Input: part model. Units: mm. Frame: model coordinates. Face numbers are marked on the shaded views. A direction names the side the tool comes from. Coordinates: 2 decimals unless noted, no trailing zeros. Order: outer loops, then holes, each group sorted by start corner. A loop starts at its lowest first (then second) coordinate and runs counter-clockwise, first axis right, second up. Notation, with made-up numbers: (-9, -18) -> (18, -18) arc R28 cw to (18, 20) -> close; hole circle Ø2 at (4.5, 7.25). An arc over 180 degrees is marked (long way). Answer as CSV lines item,"result".
from build123d import *

# Parameters (mm, degrees)
BOSS_EXTRU_1_START             = 0.6
ESQUISSE1_R                    = 47
ESQUISSE1_R_2                  = 20
BOSS_EXTRU_1_DEPTH             = 3
ESQUISSE2_R                    = 34.05
ESQUISSE2_R_2                  = 31.05
BOSS_EXTRU_2_DEPTH             = 8
CHANFREIN1_SIZE                = 0.5
TROU_TARAUD_M4X0_71_AT_2_COUNT = 2
TROU_TARAUD_M4X0_71_AT_2_PITCH = 12.5
TROU_TARAUD_M4X0_71_AT_3_COUNT = 2
TROU_TARAUD_M4X0_71_AT_3_PITCH = 82
TROU_TARAUD_M4X0_71_AT_4_COUNT = 2
TROU_TARAUD_M4X0_71_AT_4_PITCH = 82.947272408
TROU_TARAUD_M4X0_71_AT_5_COUNT = 2
TROU_TARAUD_M4X0_71_AT_5_PITCH = 49.143921292
TROU_TARAUD_M4X0_71_AT_6_COUNT = 2
TROU_TARAUD_M4X0_71_AT_6_PITCH = 58.652578801
TROU_TARAUD_M4X0_71_AT_7_COUNT = 2
TROU_TARAUD_M4X0_71_AT_7_PITCH = 66.821590822
TROU_TARAUD_M4X0_71_AT_8_COUNT = 2
TROU_TARAUD_M4X0_71_AT_8_PITCH = 58.652578801
TROU_TARAUD_M6X1_01_AT_2_COUNT = 2
TROU_TARAUD_M6X1_01_AT_2_PITCH = 20.705523608
TROU_TARAUD_M6X1_01_AT_3_COUNT = 2
TROU_TARAUD_M6X1_01_AT_3_PITCH = 56.568542495
TROU_TARAUD_M6X1_01_AT_4_COUNT = 2
TROU_TARAUD_M6X1_01_AT_4_PITCH = 69.282032303
TROU_TARAUD_M6X1_01_AT_5_COUNT = 2
TROU_TARAUD_M6X1_01_AT_5_PITCH = 80
TROU_TARAUD_M6X1_01_AT_6_COUNT = 2
TROU_TARAUD_M6X1_01_AT_6_PITCH = 77.274066103
TROU_TARAUD_M6X1_01_AT_7_COUNT = 2
TROU_TARAUD_M6X1_01_AT_7_PITCH = 56.568542495
TROU_TARAUD_M6X1_01_AT_8_COUNT = 2
TROU_TARAUD_M6X1_01_AT_8_PITCH = 40
D_GAGEMENT_M31_D               = 3.4


with BuildPart() as part:
    # Esquisse1 → Boss.-Extru.1 (new body)
    with BuildSketch(Plane.XY.offset(BOSS_EXTRU_1_START)):
        Circle(ESQUISSE1_R)
        Circle(ESQUISSE1_R_2, mode=Mode.SUBTRACT)
    extrude(amount=BOSS_EXTRU_1_DEPTH)

    # Esquisse2 → Boss.-Extru.2 (add)
    with BuildSketch(Plane(origin=(0, 0, 0.6), x_dir=(-1, 0, 0), z_dir=(0, 0, -1))):
        with Locations(Location((0, 0, 0), (0, 0, 180))):
            Circle(ESQUISSE2_R)
        Circle(ESQUISSE2_R_2, mode=Mode.SUBTRACT)
    extrude(amount=BOSS_EXTRU_2_DEPTH)

    # Chanfrein1
    chanfrein1_edges = [part.edges().sort_by_distance(p)[0] for p in [
        (-34.05, 0, -7.4),
        (31.05, 0, -7.4),
    ]]
    chamfer(chanfrein1_edges, length=CHANFREIN1_SIZE)

    # Esquisse15 → Trou taraudé M4x0.71 (revolve, cut)
    with BuildSketch(Plane(origin=(6.25, 41, 3.6), x_dir=(0, -1, 0), z_dir=(1, 0, 0))):
        Polygon((0, 0), (0, 3), (2.125, 3), (1.65, 2.525), (1.65, 0.475), (2.125, 0), align=None)
    trou_taraud_m4x0_71 = revolve(axis=Axis((6.25, 41, 9.95), (0, 0, -1)), mode=Mode.SUBTRACT)

    # Trou taraudé M4x0.71 at 2: Trou taraudé M4x0.71 ×2
    with Locations(*[(-i * TROU_TARAUD_M4X0_71_AT_2_PITCH, 0, 0) for i in range(1, TROU_TARAUD_M4X0_71_AT_2_COUNT)]):
        add(trou_taraud_m4x0_71, mode=Mode.SUBTRACT)

    # Trou taraudé M4x0.71 at 3: Trou taraudé M4x0.71 ×2
    with Locations(*[(0, -i * TROU_TARAUD_M4X0_71_AT_3_PITCH, 0) for i in range(1, TROU_TARAUD_M4X0_71_AT_3_COUNT)]):
        add(trou_taraud_m4x0_71, mode=Mode.SUBTRACT)

    # Trou taraudé M4x0.71 at 4: Trou taraudé M4x0.71 ×2
    with Locations(*[Vector(-0.15069814397812628, -0.9885798244965087, 0) * (i * TROU_TARAUD_M4X0_71_AT_4_PITCH) for i in range(1, TROU_TARAUD_M4X0_71_AT_4_COUNT)]):
        add(trou_taraud_m4x0_71, mode=Mode.SUBTRACT)

    # Trou taraudé M4x0.71 at 5: Trou taraudé M4x0.71 ×2
    with Locations(*[Vector(0.7071067811865477, -0.7071067811865474, 0) * (i * TROU_TARAUD_M4X0_71_AT_5_PITCH) for i in range(1, TROU_TARAUD_M4X0_71_AT_5_COUNT)]):
        add(trou_taraud_m4x0_71, mode=Mode.SUBTRACT)

    # Trou taraudé M4x0.71 at 6: Trou taraudé M4x0.71 ×2
    with Locations(*[Vector(0.5924718181265287, -0.8055911771648481, 0) * (i * TROU_TARAUD_M4X0_71_AT_6_PITCH) for i in range(1, TROU_TARAUD_M4X0_71_AT_6_COUNT)]):
        add(trou_taraud_m4x0_71, mode=Mode.SUBTRACT)

    # Trou taraudé M4x0.71 at 7: Trou taraudé M4x0.71 ×2
    with Locations(*[Vector(-0.7071067811865475, -0.7071067811865477, 0) * (i * TROU_TARAUD_M4X0_71_AT_7_PITCH) for i in range(1, TROU_TARAUD_M4X0_71_AT_7_COUNT)]):
        add(trou_taraud_m4x0_71, mode=Mode.SUBTRACT)

    # Trou taraudé M4x0.71 at 8: Trou taraudé M4x0.71 ×2
    with Locations(*[Vector(-0.8055911771648481, -0.5924718181265287, 0) * (i * TROU_TARAUD_M4X0_71_AT_8_PITCH) for i in range(1, TROU_TARAUD_M4X0_71_AT_8_COUNT)]):
        add(trou_taraud_m4x0_71, mode=Mode.SUBTRACT)

    # Esquisse17 → Trou taraudé M6x1.01 (revolve, cut)
    with BuildSketch(Plane(origin=(34.641016151, 20, 0.6), x_dir=(0, 1, 0), z_dir=(1, 0, 0))):
        Polygon((0, 0), (0, 3), (3.125, 3), (2.5, 2.375), (2.5, 0.625), (3.125, 0), align=None)
    trou_taraud_m6x1_01 = revolve(axis=Axis((34.641016151, 20, -5.75), (0, 0, 1)), mode=Mode.SUBTRACT)

    # Trou taraudé M6x1.01 at 2: Trou taraudé M6x1.01 ×2
    with Locations(*[Vector(-0.7071067811865414, 0.7071067811865538, 0) * (i * TROU_TARAUD_M6X1_01_AT_2_PITCH) for i in range(1, TROU_TARAUD_M6X1_01_AT_2_COUNT)]):
        add(trou_taraud_m6x1_01, mode=Mode.SUBTRACT)

    # Trou taraudé M6x1.01 at 3: Trou taraudé M6x1.01 ×2
    with Locations(*[Vector(-0.9659258262890666, 0.25881904510252685, 0) * (i * TROU_TARAUD_M6X1_01_AT_3_PITCH) for i in range(1, TROU_TARAUD_M6X1_01_AT_3_COUNT)]):
        add(trou_taraud_m6x1_01, mode=Mode.SUBTRACT)

    # Trou taraudé M6x1.01 at 4: Trou taraudé M6x1.01 ×2
    with Locations(*[(-i * TROU_TARAUD_M6X1_01_AT_4_PITCH, 0, 0) for i in range(1, TROU_TARAUD_M6X1_01_AT_4_COUNT)]):
        add(trou_taraud_m6x1_01, mode=Mode.SUBTRACT)

    # Trou taraudé M6x1.01 at 5: Trou taraudé M6x1.01 ×2
    with Locations(*[Vector(-0.8660254037844417, -0.49999999999999467, 0) * (i * TROU_TARAUD_M6X1_01_AT_5_PITCH) for i in range(1, TROU_TARAUD_M6X1_01_AT_5_COUNT)]):
        add(trou_taraud_m6x1_01, mode=Mode.SUBTRACT)

    # Trou taraudé M6x1.01 at 6: Trou taraudé M6x1.01 ×2
    with Locations(*[Vector(-0.7071067811865456, -0.7071067811865496, 0) * (i * TROU_TARAUD_M6X1_01_AT_6_PITCH) for i in range(1, TROU_TARAUD_M6X1_01_AT_6_COUNT)]):
        add(trou_taraud_m6x1_01, mode=Mode.SUBTRACT)

    # Trou taraudé M6x1.01 at 7: Trou taraudé M6x1.01 ×2
    with Locations(*[Vector(-0.25881904510252607, -0.9659258262890669, 0) * (i * TROU_TARAUD_M6X1_01_AT_7_PITCH) for i in range(1, TROU_TARAUD_M6X1_01_AT_7_COUNT)]):
        add(trou_taraud_m6x1_01, mode=Mode.SUBTRACT)

    # Trou taraudé M6x1.01 at 8: Trou taraudé M6x1.01 ×2
    with Locations(*[(0, -i * TROU_TARAUD_M6X1_01_AT_8_PITCH, 0) for i in range(1, TROU_TARAUD_M6X1_01_AT_8_COUNT)]):
        add(trou_taraud_m6x1_01, mode=Mode.SUBTRACT)

    # Dégagement M31 (through all)
    with Locations(Plane(origin=(27.25, 0, 3.6), x_dir=(1, 0, 0), z_dir=(0, 0, 1))):
        with Locations((0, 0), (-13.625, 23.599192253), (-40.875, 23.599192253), (-54.5, 0), (-40.875, -23.599192253), (-13.625, -23.599192253)):
            Hole(D_GAGEMENT_M31_D / 2)


solid = part.part
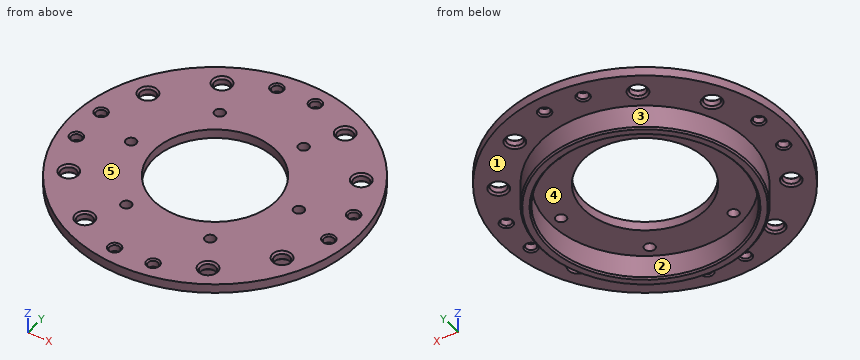
1. Mould query, pull axis Y, two halves, no side actions, for the marked faces 1, 2 and 3. Classes: released by +Y, released by -Y, zero draft, split by the parting line, or undercut.
Findings:
face 1,"zero draft"
face 2,"undercut"
face 3,"split by the parting line"
2. Cut plane A-A (y = 0). Return the cut outline in (x, z), plus the area to 3 significant figures.
Findings:
outline,"(-47, 0.6) -> (-34.05, 0.6) -> (-34.05, -6.9) -> (-33.55, -7.4) -> (-31.55, -7.4) -> (-31.05, -6.9) -> (-31.05, 0.6) -> (-28.95, 0.6) -> (-28.95, 3.6) -> (-47, 3.6) -> close; (-25.55, 0.6) -> (-20, 0.6) -> (-20, 3.6) -> (-25.55, 3.6) -> close; (20, 0.6) -> (25.55, 0.6) -> (25.55, 3.6) -> (20, 3.6) -> close; (28.95, 0.6) -> (31.05, 0.6) -> (31.05, -6.9) -> (31.55, -7.4) -> (33.55, -7.4) -> (34.05, -6.9) -> (34.05, 0.6) -> (47, 0.6) -> (47, 3.6) -> (28.95, 3.6) -> close"
area,"189 mm2"
3. Reachability of the marked faces 4 and 5 from +Z, -Z, +X, -X, +Y, -Y: full face, straight path, thin tool, end or side. Return the list, or none.
Findings:
face 4,"-Z"
face 5,"+Z, +X, -X, +Y, -Y"
4. Contact query for flat-ended pins moving along their axis: pin 1 (4 mm diameter, centred on x = -6.25, y = -41, fed in from +Z) (3 decimals); pin 2 (4 mm diameter, centred on x = 41, y = 6.25, fed in from -Z) (3 decimals); pin 3 (1.5 mm diameter, centred on x = -29.5, z = 1.5, fed in from +Y); pin 4 (4 mm diameter, centred on x = 27.25, y = 0, fed in from +Z). Output: stop coordinate, or through.
Findings:
pin 1,"stops at z = 3.475"
pin 2,"stops at z = 0.725"
pin 3,"stops at y = 37.18"
pin 4,"stops at z = 3.6"
5. Cut plane B-B (x = -41). Return the cut outline in (y, z) (3 decimals), plus the area to 3 significant figures.
Findings:
outline,"(-22.978, 0.6) -> (-8.375, 0.6) -> (-7.9, 1.075) -> (-7.9, 3.125) -> (-8.375, 3.6) -> (-22.978, 3.6) -> close; (-4.6, 1.075) -> (-4.125, 0.6) -> (4.125, 0.6) -> (4.6, 1.075) -> (4.6, 3.125) -> (4.125, 3.6) -> (-4.125, 3.6) -> (-4.6, 3.125) -> close; (7.9, 1.075) -> (8.375, 0.6) -> (22.978, 0.6) -> (22.978, 3.6) -> (8.375, 3.6) -> (7.9, 3.125) -> close"
area,"117 mm2"
6. Cut plane C-C (z = -3). Return the cut outline in (x, y), plus the area to 3 significant figures.
Findings:
outline,"circle Ø68.1 at (0, 0); hole circle Ø62.1 at (0, 0)"
area,"614 mm2"
7. Ray query, line 1 along X through (y, z) = (41, 2.3); line 2 along X through (y, z) = (18, 3); line 3 along Y through (x, z) = (6.25, 2.35). Return the intervals inside material, ascending.
Findings:
line 1,"x = -22.98 to -7.9, -4.6 to 4.6, 7.9 to 22.98"
line 2,"x = -43.42 to -36.18, -33.1 to -8.72, 8.72 to 33.1, 36.18 to 43.42"
line 3,"y = -46.58 to -42.65, -39.35 to -19, 19 to 39.35, 42.65 to 46.58"
